Geometry: final body of the model. Coordinates: model frame, mm. Face numbers are marked on the shaded views. A direction names the side the tool comes from. Give positions to 0.01 mm unless a question says otherwise; leave off trailing zeros. Write each loop counter-clockwise with the first axis right and the second up, starting at its lowest first coordinate (ties: lowest second). Pieces come first, ordered by that corner, then holes. Notation, with made-up numbers: (18, 31.25) -> (30, 31.25) arc R12 cw to (30, 47.25) -> close; hole circle Ø8 at (-18.5, 59). An arc over 180 degrees is marked (long way). Answer as a JSON object with one key per item and string values. Group by question number.
(1) Section query D-D on z = -9. Output: boundary loops of the cut face in (x, y).
(2) Section query B-B on y = 5. Output: boundary loops of the cut face in (x, z).
(3) Set-up query: the marked faces 1, 2 and 3. Return all of +Z, -Z, +X, -X, +Y, -Y with unobstructed straight access to the full face (end or side cutting, diameter ignored); none if empty.
(4) Section query C-C on y = 21. Output: boundary loops of the cut face in (x, z).
(5) Section query A-A on z = 0. Output: boundary loops of the cut face in (x, y), plus the area to 3 significant figures.
(6) Material intervals for probe 1 along Y at (x, z) = (5, -6); probe 2 along Z at (x, y) = (4.75, 5); probe 3 along Z at (x, y) = (-1.25, 5), sorted ascending.
(7) Contact query for flat-ended pins moving along their axis: pin 1 Ø4 at (y, z) = (5, 0) entering from +X; pin 2 Ø10 at (x, y) = (0, 21) entering from +Z; pin 3 Ø8 at (y, z) = (5.5, -8) entering from +X. Output: stop coordinate, or through.
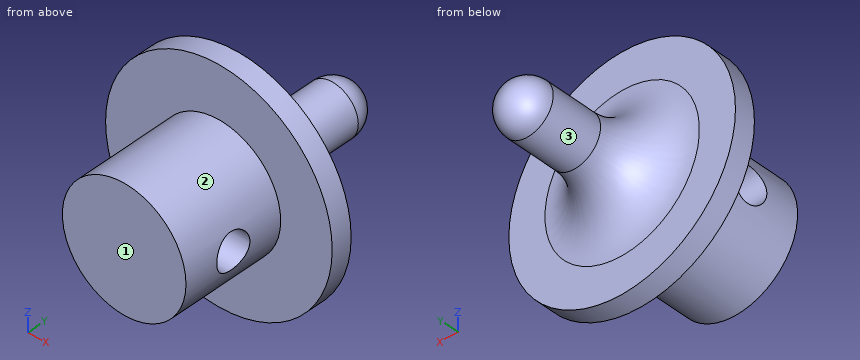
from build123d import *

# Parameters (mm, degrees)
SKETCH1_R               = 6
BOSS_EXTRUDE1_DEPTH     = 10
SKETCH2_R               = 11
BOSS_EXTRUDE2_DEPTH     = 2
FILLET1_R               = 5
SKETCH5_R               = 1.75
CUT_EXTRUDE1_DEPTH      = 12
CUT_EXTRUDE1_DEPTH_BACK = 12


with BuildPart() as part:
    # Sketch1 → Boss-Extrude1 (new body)
    with BuildSketch(Plane(origin=(0, 0, 0), x_dir=(1, 0, 0), z_dir=(0, 1, 0))):
        Circle(SKETCH1_R)
    extrude(amount=BOSS_EXTRUDE1_DEPTH)

    # Sketch2 → Boss-Extrude2 (add)
    with BuildSketch(Plane(origin=(0, 10, 0), x_dir=(1, 0, 0), z_dir=(0, 1, 0))):
        Circle(SKETCH2_R)
    extrude(amount=BOSS_EXTRUDE2_DEPTH)

    # Sketch3 → Revolve1 (revolve)
    with BuildSketch(Plane(origin=(0, 0, 0), x_dir=(0, 0, -1), z_dir=(1, 0, 0))):
        with BuildLine():
            Line((0, 12), (-2.5, 12))
            Line((-2.5, 12), (-2.5, 22))
            ThreePointArc((-2.5, 22), (-1.767766953, 23.767766953), (0, 24.5))
            Line((0, 24.5), (0, 12))
        make_face()
    revolve(axis=Axis((0, 24.5, 0), (0, -1, 0)))

    # Fillet1
    fillet1_edges = [part.edges().sort_by_distance(p)[0] for p in [
        (0, 12, -2.5),
    ]]
    fillet(fillet1_edges, radius=FILLET1_R)

    # Sketch5 → Cut-Extrude1 (cut, two sides)
    with BuildSketch(Plane(origin=(0, 0, 0), x_dir=(0, 0, -1), z_dir=(1, 0, 0))) as cut_extrude1_sk:
        with Locations((0, 5)):
            Circle(SKETCH5_R)
    extrude(amount=CUT_EXTRUDE1_DEPTH, mode=Mode.SUBTRACT)
    extrude(cut_extrude1_sk.sketch, amount=-CUT_EXTRUDE1_DEPTH_BACK, mode=Mode.SUBTRACT)


solid = part.part
Answer list:
{
 "1": {"outline": "(-6.32, 10) -> (6.32, 10) -> (6.32, 12) -> (-6.32, 12) -> close"},
 "2": {"outline": "(-5.74, -1.75) arc R6 ccw to (5.74, -1.75) -> close; (-5.74, 1.75) -> (5.74, 1.75) arc R6 ccw to start"},
 "3": {"face 1": "+Z, -Z, +X, -X, -Y", "face 2": "-Y", "face 3": "+Y"},
 "4": {"outline": "circle Ø5 at (0, 0)"},
 "5": {"outline": "(-11, 10) -> (-6, 10) -> (-6, 6.75) -> (6, 6.75) -> (6, 10) -> (11, 10) -> (11, 12) -> (7.5, 12) arc R5 cw to (2.5, 17) -> (2.5, 22) arc R2.5 ccw to (-2.5, 22) -> (-2.5, 17) arc R5 cw to (-7.5, 12) -> (-11, 12) -> close; (-6, 0) -> (6, 0) -> (6, 3.25) -> (-6, 3.25) -> close", "area": "193 mm2"},
 "6": {"probe 1": "10 to 12", "probe 2": "-3.67 to -1.75, 1.75 to 3.67", "probe 3": "-5.87 to -1.75, 1.75 to 5.87"},
 "7": {"pin 1": "x = 6", "pin 2": "z = 2.6", "pin 3": "x = 4.47"}
}
